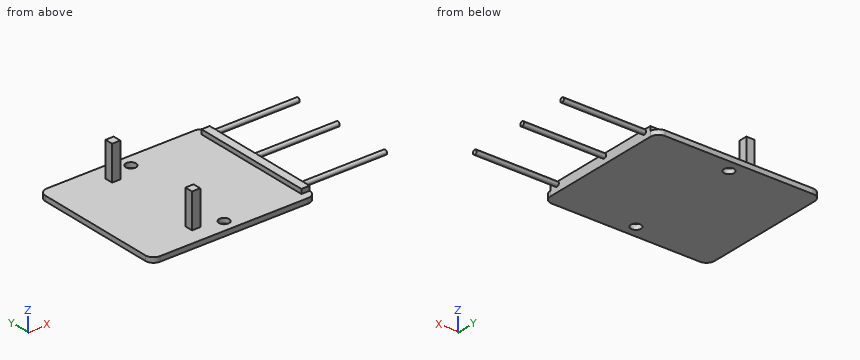
```python
from build123d import *

# Parameters (mm, degrees)
F1_DEPTH = 1.5494
F2_R     = 1.5875
F3_DEPTH = 25.4
F4_W     = 2.54
F4_H     = 2.54
F5_DEPTH = 10.668
F7_W     = 2.54
F7_H     = 38.1
F8_DEPTH = 1.397
F9_DEPTH = 25.4


with BuildPart() as f1:
    # F0 (on Top) → F1 (new body)
    with BuildSketch(Plane.XY):
        with BuildLine():
            ThreePointArc((0, 2.54), (0.743949, 0.743949), (2.54, 0))
            Line((2.54, 0), (48.26, 0))
            ThreePointArc((48.26, 0), (50.056051, 0.743949), (50.8, 2.54))
            Line((50.8, 2.54), (50.8, 40.64))
            ThreePointArc((50.8, 40.64), (50.056051, 42.436051), (48.26, 43.18))
            Line((48.26, 43.18), (2.54, 43.18))
            ThreePointArc((2.54, 43.18), (0.743949, 42.436051), (0, 40.64))
            Line((0, 40.64), (0, 2.54))
        make_face()
    extrude(amount=F1_DEPTH)

    # F2 (on face) → F3 (cut)
    with BuildSketch(Plane.XY.offset(1.5494)):
        with Locations((25.4, 39.37)):
            Circle(F2_R)
        with Locations((25.4, 3.81)):
            Circle(F2_R)
    extrude(amount=-F3_DEPTH, mode=Mode.SUBTRACT)

    # F4 (on face) → F5 (join)
    with BuildSketch(Plane.XY.offset(1.5494)):
        with Locations((17.78, 36.83)):
            Rectangle(F4_W, F4_H)
        with Locations((17.78, 6.35)):
            Rectangle(F4_W, F4_H)
    extrude(amount=F5_DEPTH)

    # F7 (on face) → F8 (join)
    with BuildSketch(Plane.XY.offset(1.5494)):
        with Locations((49.53, 21.59)):
            Rectangle(F7_W, F7_H)
    extrude(amount=F8_DEPTH)

    # F6 (on face) → F9 (join)
    with BuildSketch(Plane.YZ.offset(50.8)):
        with BuildLine():
            ThreePointArc((5.08, 1.5494), (5.573914, 1.753986), (5.7785, 2.2479))
            ThreePointArc((5.7785, 2.2479), (4.586086, 2.741814), (5.08, 1.5494))
        make_face()
        with BuildLine():
            ThreePointArc((23.8125, 2.2479), (22.620086, 2.741814), (23.114, 1.5494))
            ThreePointArc((23.114, 1.5494), (23.607914, 1.753986), (23.8125, 2.2479))
        make_face()
        with BuildLine():
            ThreePointArc((39.0525, 2.2479), (37.860086, 2.741814), (38.354, 1.5494))
            ThreePointArc((38.354, 1.5494), (38.847914, 1.753986), (39.0525, 2.2479))
        make_face()
    extrude(amount=F9_DEPTH)


solid = f1.part
```
Here's how the part is built. I have some questions about the finished solid (model axes, mm). Give positions to 0.01 mm unless a question says otherwise; leave off trailing zeros. Write each loop counter-clockwise with the first axis right and the second up, starting at its lowest first coordinate (ties: lowest second). Pieces come first, ordered by that corner, then holes. Notation, with made-up numbers: M 76,49 L 82,49 A21 ccw 82,84 Z; hole C -7,56 d10. An arc over 180 degrees is marked long. Put each result on its own line as item: value. Start each with the question number.
Item 1: If we section it at B-B, the plane z = 10.5: Write out the boundary of the cut face in (x, y), then the cut area to 3 significant figures.
Item 2: If we section it at A-A, the plane x = 25.4: Write out the boundary of the cut face in (y, z).
Item 3: Will these pins go through, and if not, where does the flat tip stop? pin 1 (4 mm diameter, centred on x = 66.5, y = 5, fed in from +Z); pin 2 (6 mm diameter, centred on x = 29, y = 6, fed in from +Z); pin 3 (3 mm diameter, centred on x = 17, z = 4.5, fed in from -Y); pin 4 (2 mm diameter, centred on x = 37.5, y = 8.5, fed in from -Z).
Item 4: If we section it at D-D, the plane x = 57.5: Write out the boundary of the cut face in (y, z).
Item 5: I need wall thicknesses on L1, parallel to Y at x = 25.4, z = 0.3; L2, parallel to X at y = 4, z = 1.25; L3, parallel to Z at x = 14.5, y = 16. Which ranges of each line are inside material? Lowest first, please. Write a range as from..to.
Item 6: If we section it at C-C, the plane y = 31.5: Write out the boundary of the cut face in (x, z).
Values:
1. outline: M 16.51,5.08 L 19.05,5.08 L 19.05,7.62 L 16.51,7.62 Z; M 16.51,35.56 L 19.05,35.56 L 19.05,38.1 L 16.51,38.1 Z
1. area: 12.9 mm²
2. outline: M 0,0 L 2.22,0 L 2.22,1.55 L 0,1.55 Z; M 5.4,0 L 37.78,0 L 37.78,1.55 L 5.4,1.55 Z; M 40.96,0 L 43.18,0 L 43.18,1.55 L 40.96,1.55 Z
3. pin 1: z = 2.95
3. pin 2: z = 1.55
3. pin 3: y = 5.08
3. pin 4: z = 0
4. outline: C 5.08,2.25 d1.4; C 23.11,2.25 d1.4; C 38.35,2.25 d1.4
5. L1: 0..2.22, 5.4..37.78, 40.96..43.18
5. L2: 0..23.82, 26.98..50.8
5. L3: 0..1.55
6. outline: M 0,0 L 50.8,0 L 50.8,2.95 L 48.26,2.95 L 48.26,1.55 L 0,1.55 Z
